Autodesk Inventor part; units mm, degrees
ref_plane "YZ Plane" through (0, 0, 0) normal (1, 0, 0) x (0, 1, 0)
ref_plane "XZ Plane" through (0, 0, 0) normal (0, 1, 0) x (-1, 0, 0)
ref_plane "XY Plane" through (0, 0, 0) normal (0, 0, 1) x (1, 0, 0)
sketch "スケッチ1" plane through (0, 0, 0) normal (1, 0, 0) x (0, 1, 0)
  line L0 (0, 0) -> (1, 0) construction
  line L1 (1.9, 0) -> (1.9, 1.75)
  line L2 (1.65, 2) -> (0.866, 2)
  line L3 (0, 2) -> (0, 1.5) construction
  line L4 (1, 0) -> (1, -6)
  line L5 (1, -6) -> (0, -6)
  line L6 (0, -6) -> (0, 0)
  line L7 (1, 0) -> (1.9, 0)
  line L8 (0.866, 2) -> (0.433, 1.25) construction
  line L9 (0.433, 1.25) -> (-0.433, 1.25) construction
  line L10 (-0.433, 1.25) -> (-0.866, 2) construction
  line L11 (-0.866, 2) -> (-0.433, 2.75) construction
  line L12 (-0.433, 2.75) -> (0.433, 2.75) construction
  line L13 (0.433, 2.75) -> (0.866, 2) construction
  line L14 (0.866, 2) -> (0, 1.5)
  line L15 (0.866, 2) -> (0, 2) construction
  line L16 (0, 1.5) -> (0, 0)
  arc A0 (1.9, 1.75) -> (1.65, 2) centre (1.65, 1.75) ccw
  dimension "d0" = 1.5
  dimension "d1" = 3.8
  dimension "d2" = 2
  dimension "d3" = 6
  dimension "d4" = 2
  dimension "d6" = 0.25
  dimension "d11" = 30
revolve "回転1" add sketch "スケッチ1" angle 360 about axis through (0, 0, 1.5) along (0, 0, -1)
sketch "スケッチ2" plane through (0, 0, 2) normal (0, 0, 1) x (1, 0, 0)
  line L0 (0.866, 0) -> (0.433, -0.75)
  line L1 (0.433, -0.75) -> (-0.433, -0.75)
  line L2 (-0.433, -0.75) -> (-0.866, 0)
  line L3 (-0.866, 0) -> (-0.433, 0.75)
  line L4 (-0.433, 0.75) -> (0.433, 0.75)
  line L5 (0.433, 0.75) -> (0.866, 0)
  point P0 (0, 0)
  point P1 (0, 0)
  dimension "d8" = 1.5
extrude "押し出し1" cut sketch "スケッチ2" against normal blind 1
chamfer "面取り1" distance 0.25 angle 45 1 edges at (0, -1, -6)
properties part number "10_050_CAP_BOLT_M2X6_R1" material "鋼、炭素鋼"
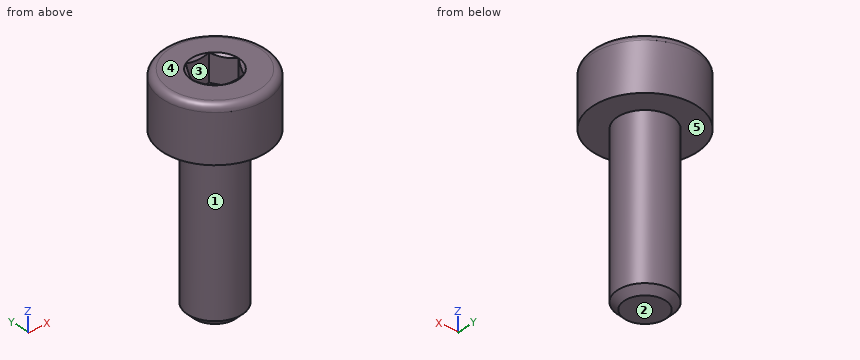
Work out the finished part from the listing and answer in its coordinate system (mm). Face numbers are marked on the shaded views. A direction names the side the tool comes from. Give positions to 0.01 mm unless a question says otherwise; leave off trailing zeros. Order: outer loops, then holes, each group sorted by start corner. A loop starts at its lowest first (then second) coordinate and runs counter-clockwise, first axis right, second up. Notation, with made-up numbers: (20, 84.25) - (52, 84.25) arc R12 ccw to (52, 102.25) - close; hole circle Ø8 at (-31, 37.5). An arc over 180 degrees is marked (long way). One line per item, written item: value. Start each with the question number.
1. Each of these flat-tipped pins is pushed along its axis until it touches: pin 1 Ø1.2 at (x, y) = (0, 0) entering from +Z; pin 2 Ø1.5 at (x, y) = (1, 0) entering from -Z. Where does it stop, or does it pass through?
2. For a pull along Y with two mould halves and no side action, classify the marked faces 1, 2 and 3 as released by +Y, released by -Y, zero draft, split by the parting line, or undercut.
3. Section A-A, the plane x = 0 is taken. Write down the section's boundary in (y, z), then the cut area to 3 significant figures.
4. Which of the six approach directions +Z, -Z, +X, -X, +Y, -Y give full straight-line access (tool end or side, diameter ignored) to the marked faces 4 and 5?
5. Section B-B, the plane z = -2 is taken. Write down the section's boundary in (x, y), then the cut area to 3 significant figures.
6. Consider line 1 (Y direction, x = -0.35, z = 1.25); line 2 (X direction, y = 0.9, z = -0.75); line 3 (Z direction, x = 0.45, y = -1.1). Determine where each line is inside the solid, lowest interval first.
Filled sheet:
1. pin 1: z = 1
1. pin 2: z = -6
2. face 1: split by the parting line
2. face 2: zero draft
2. face 3: undercut
3. outline: (-1.9, 0) - (-1, 0) - (-1, -5.75) - (-0.75, -6) - (0.75, -6) - (1, -5.75) - (1, 0) - (1.9, 0) - (1.9, 1.75) arc R0.25 ccw to (1.65, 2) - (0.87, 2) - (0.75, 1.93) - (0.75, 1) - (-0.75, 1) - (-0.75, 1.93) - (-0.87, 2) - (-1.65, 2) arc R0.25 ccw to (-1.9, 1.75) - close
3. area: 18.0 mm²
4. face 4: +Z, +X, -X, +Y, -Y
4. face 5: -Z
5. outline: circle Ø2 at (0, 0)
5. area: 3.14 mm²
6. line 1: -1.87 to -0.75, 0.75 to 1.87
6. line 2: -0.44 to 0.44
6. line 3: 0 to 2
